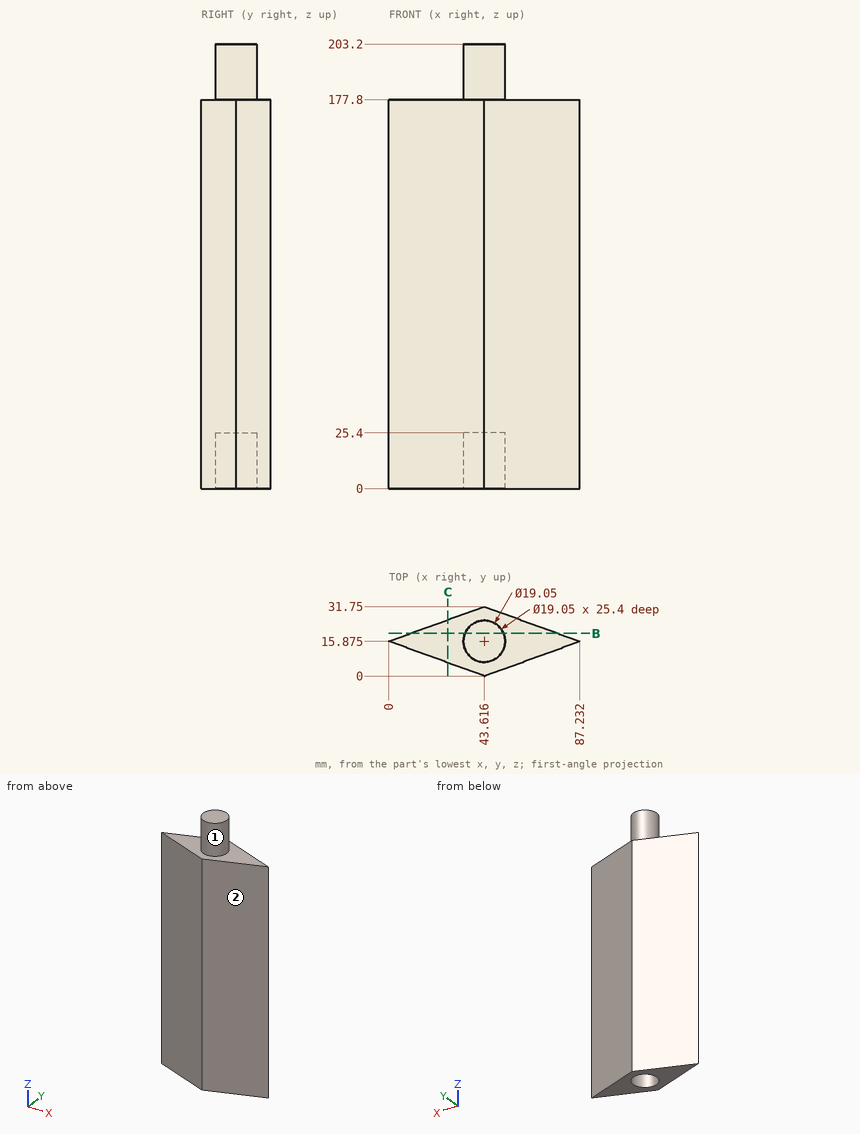
Geometry check sheet. Reference: drawing and pictorial views, mm from the part's lowest x, y, z. A direction names the side the tool comes from. Give positions to 0.01 mm unless a question says otherwise; leave off trailing zeros. Loops run counter-clockwise (first coordinate to the right, second up) from the corner with the lowest first, then second, coordinate; pieces in that order, holes last. Notation, with made-up numbers: (-35, 65.25) - (17, 65.25) arc R35 cw to (17, 102.25) - close; hole circle Ø1 at (59.5, 52). An arc over 180 degrees is marked (long way). One line per question, with ' | ' between items. Start each with the question number.
1. Cross-section at B-B, the plane y = 19.5. Enter the section's corners in (x, z) (1 decimal).
2. Set-up check for the marked faces 1 and 2: record each of +Z, -Z, +X, -X, +Y, -Y from which the full face is reachable in a straight line by a thin tool's end or side.
3. Cross-section at C-C, the plane x = 27. Enter the section's corners in (y, z).
4. Material ranges on line 1 along Z through (x, y) = (75.5, 19.5); line 2 along Y through (x, z) = (42.5, 14) (1 decimal); line 3 along Y through (x, z) = (82, 26.5), recorded low to high. Write a range as [from, to].
5. Gauge pin test, flat ends, axial feed: pin 1 Ø2 at (x, y) = (57.5, 20) entering from +Z; pin 2 Ø5 at (x, z) = (63, 169) entering from +Y (1 decimal); pin 3 Ø9.5 at (x, y) = (44, 18) entering from -Z. Record the tip position at first contact, or that the pin passes through.
Check result:
1) outline: (10, 0) - (34.8, 0) - (34.8, 25.4) - (52.4, 25.4) - (52.4, 0) - (77.3, 0) - (77.3, 177.8) - (52.4, 177.8) - (52.4, 203.2) - (34.8, 203.2) - (34.8, 177.8) - (10, 177.8) - close
2) face 1: +Z | face 2: +Z, -Z, +X, -Y
3) outline: (6.05, 0) - (25.7, 0) - (25.7, 177.8) - (6.05, 177.8) - close
4) line 1: z = [0, 177.8] | line 2: y = [0.4, 6.4], [25.3, 31.3] | line 3: y = [13.97, 17.78]
5) pin 1: stops at z = 177.8 | pin 2: stops at y = 25.6 | pin 3: stops at z = 25.4
